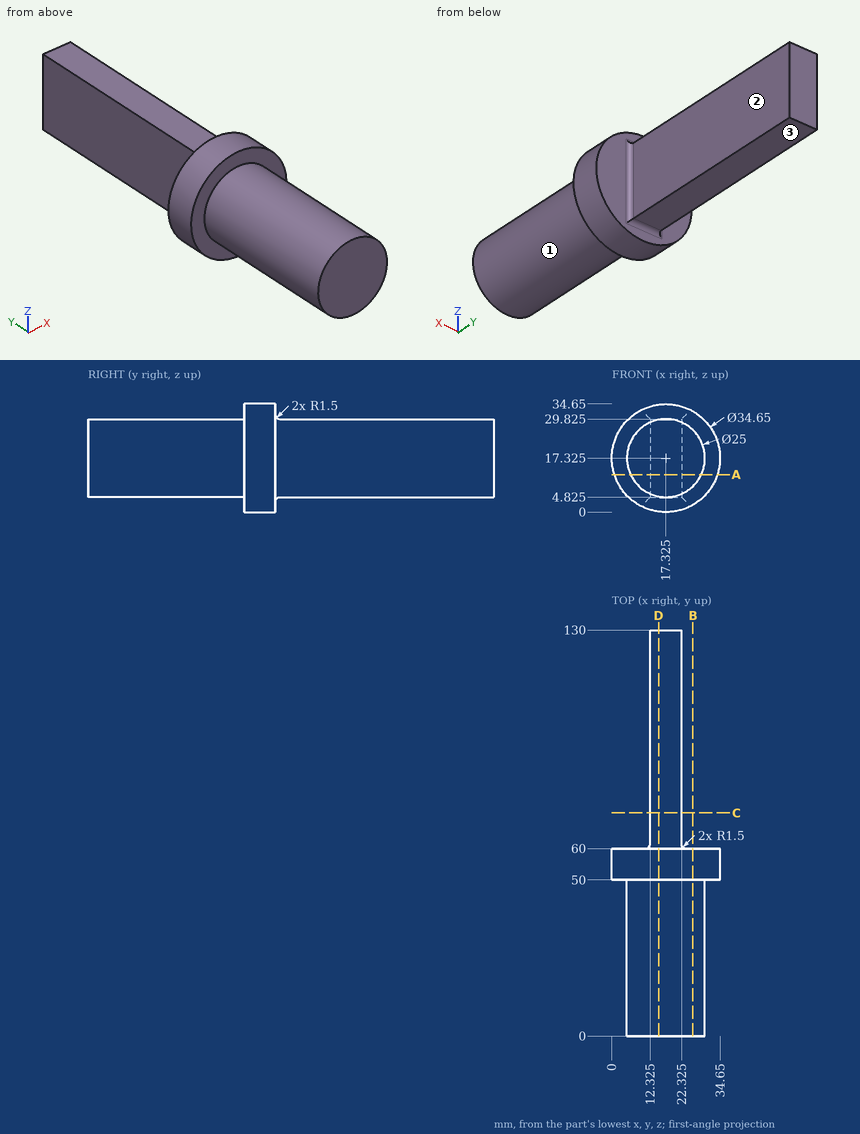
For this review, use the dimensioned drawing (mm, ordinates from the lowest corner) and the shaded views. A direction names the side the tool comes from. Round coordinates to 2 decimals unless told otherwise and drop trailing zeros. Loops run counter-clockwise (first coordinate to the right, second up) from the corner with the lowest first, then second, coordinate; pieces in that order, holes last. Notation, with made-up numbers: M 37,50.25 L 75,50.25 A24 ccw 75,81.25 Z; hole C -2,43 d1. An arc over 180 degrees is marked long. Answer as CSV lines item,"result".
1. We need section D-D (x = 15). Give the boundary of the cut face in (y, z) (3 decimals), plus the area to 3 significant figures.
Outcome:
outline,"M 0,5.043 L 50,5.043 L 50,0.157 L 60,0.157 L 60,3.325 A1.5 cw 61.5,4.825 L 130,4.825 L 130,29.825 L 61.5,29.825 A1.5 cw 60,31.325 L 60,34.493 L 50,34.493 L 50,29.607 L 0,29.607 Z"
area,"3,320 mm2"
2. For the marked faces 1, 2 and 3, list the 3-axis set-ups (+Z, -Z, +X, -X, +Y, -Y) from which the entire face can be reached by the end or side of a thin tool; tool diameter is ignored.
Outcome:
face 1,"-Y"
face 2,"+Z, -Z, +X, +Y"
face 3,"-Z, +X, -X, +Y"
3. To check wall thickness, follow L1, parallel to X at y = 111, z = 27 (3 decimals); L2, parallel to Y at x = 25, z = 22; L3, parallel to Z at x = 18, y = 29. State the ranges of each line that lie inside material, in increasing order. Write a range as [from, to].
Outcome:
L1,"x = [12.325, 22.325]"
L2,"y = [0, 60]"
L3,"z = [4.84, 29.81]"
4. We need section C-C (y = 71.5). Give the boundary of the cut face in (x, z) (3 decimals), plus the area to 3 significant figures.
Outcome:
outline,"M 12.325,4.825 L 22.325,4.825 L 22.325,29.825 L 12.325,29.825 Z"
area,"250 mm2"
5. We need section B-B (x = 26). Give the boundary of the cut face in (y, z).
Outcome:
outline,"M 0,8.33 L 50,8.33 L 50,2.33 L 60,2.33 L 60,32.32 L 50,32.32 L 50,26.32 L 0,26.32 Z"
6. We need section A-A (z = 12). Give the boundary of the cut face in (x, y) (3 decimals).
Outcome:
outline,"M 0.839,50 L 6.016,50 L 6.016,0 L 28.634,0 L 28.634,50 L 33.811,50 L 33.811,60 L 23.825,60 A1.5 cw 22.325,61.5 L 22.325,130 L 12.325,130 L 12.325,61.5 A1.5 cw 10.825,60 L 0.839,60 Z"
7. Insertion check: pin 1 Ø7.5 at (y, z) = (106.5, 18) entering from +X (3 decimals); pin 2 Ø5 at (x, y) = (15.5, 89) entering from +Z (3 decimals); pin 3 Ø1.5 at (y, z) = (34.5, 4) entering from +X; pin 4 Ø7.5 at (y, z) = (83, 13.5) entering from -X (3 decimals). Each pin has a flat end and moves straight along its axis. Give the tip position at first contact, or say it passes through.
Outcome:
pin 1,"stops at x = 22.325"
pin 2,"stops at z = 29.825"
pin 3,"passes through"
pin 4,"stops at x = 12.325"
